Design review of the part built by this model. Coordinates are the model's own, in mm. Face numbers are marked on the shaded views. A direction names the side the tool comes from. Coordinates: 2 decimals unless noted, no trailing zeros. Write each loop counter-clockwise with the first axis right and the second up, starting at its lowest first coordinate (ties: lowest second). Pieces come first, ordered by that corner, then holes. Notation, with made-up numbers: (-14.5, -23) - (-2.5, -23) arc R28 cw to (-2.5, 6) - close; hole circle Ø5 at (65.25, 9). An arc over 180 degrees is marked (long way). One line per item, written item: value.
from build123d import *

# Parameters (mm, degrees)
BOSS_EXTRUDE1_DEPTH      = 22
BOSS_EXTRUDE1_DEPTH_BACK = 22
SKETCH2_W                = 38
SKETCH2_H                = 20
CUT_EXTRUDE1_DEPTH       = 105.423416914
SKETCH3_W                = 7
SKETCH3_H                = 44
BOSS_EXTRUDE2_DEPTH      = 65.5
SKETCH23_R               = 5
SKETCH23_R_2             = 1.2
CUT_EXTRUDE2_DEPTH       = 111.605436123
SKETCH24_W               = 28.5
SKETCH24_H               = 34
CUT_EXTRUDE3_DEPTH       = 90.954502389
SKETCH26_R               = 1.2
SKETCH26_R_2             = 5
SKETCH26_R_3             = 1.45
CUT_EXTRUDE6_DEPTH       = 107.330263801
SKETCH27_W               = 29.7
SKETCH27_H               = 35.2
CUT_EXTRUDE8_DEPTH       = 73.137455597
SKETCH29_W               = 7
SKETCH29_H               = 35
CUT_EXTRUDE10_DEPTH      = 74.468530678
CHAMFER2_SIZE            = 5
FILLET1_START            = -23
FILLET1_DEPTH            = 46
FILLET2_R                = 10
SKETCH30_W               = 35.2
SKETCH30_H               = 20
CUT_EXTRUDE12_DEPTH      = 10


with BuildPart() as part:
    # Sketch1 → Boss-Extrude1 (new, two sides: drawn at the far end of the back side and taken through both)
    with BuildSketch(Plane.XY.offset(-BOSS_EXTRUDE1_DEPTH_BACK)):
        with BuildLine():
            Line((10.25, -60), (10.25, 0))
            ThreePointArc((10.25, 0), (0, -10.25), (-10.25, 0))
            Line((-10.25, 0), (-10.25, -60))
            Line((-10.25, -60), (-10.25, -100))
            Line((-10.25, -100), (10.25, -100))
            Line((10.25, -100), (10.25, -60))
        make_face()
        with BuildLine():
            Line((10.25, 0), (9.2, 0))
            ThreePointArc((9.2, 0), (8.816088231, -0.879772698), (7.91, -1.196620241))
            ThreePointArc((7.91, -1.196620241), (5.656854249, -5.656854249), (1.196620241, -7.91))
            ThreePointArc((1.196620241, -7.91), (1.199154762, -7.954968281), (1.2, -8))
            ThreePointArc((1.2, -8), (-0.045031719, -9.199154762), (-1.196620241, -7.91))
            ThreePointArc((-1.196620241, -7.91), (-5.656854249, -5.656854249), (-7.91, -1.196620241))
            ThreePointArc((-7.91, -1.196620241), (-8.816088231, -0.879772698), (-9.2, 0))
            Line((-9.2, 0), (-10.25, 0))
            ThreePointArc((-10.25, 0), (0, -10.25), (10.25, 0))
        make_face()
        with BuildLine():
            ThreePointArc((7.91, -1.196620241), (7.120227302, -0.816088231), (6.8, 0))
            Line((6.8, 0), (4.2, 0))
            ThreePointArc((4.2, 0), (0, -4.2), (-4.2, 0))
            Line((-4.2, 0), (-6.8, 0))
            ThreePointArc((-6.8, 0), (-7.120227302, -0.816088231), (-7.91, -1.196620241))
            ThreePointArc((-7.91, -1.196620241), (-5.656854249, -5.656854249), (-1.196620241, -7.91))
            ThreePointArc((-1.196620241, -7.91), (0, -6.8), (1.196620241, -7.91))
            ThreePointArc((1.196620241, -7.91), (5.656854249, -5.656854249), (7.91, -1.196620241))
        make_face()
        with BuildLine():
            Line((4.2, 0), (6.8, 0))
            ThreePointArc((6.8, 0), (7.120227302, 0.816088231), (7.91, 1.196620241))
            ThreePointArc((7.91, 1.196620241), (5.656854249, 5.656854249), (1.196620241, 7.91))
            ThreePointArc((1.196620241, 7.91), (0, 6.8), (-1.196620241, 7.91))
            ThreePointArc((-1.196620241, 7.91), (-5.656854249, 5.656854249), (-7.91, 1.196620241))
            ThreePointArc((-7.91, 1.196620241), (-7.120227302, 0.816088231), (-6.8, 0))
            Line((-6.8, 0), (-4.2, 0))
            ThreePointArc((-4.2, 0), (0, 4.2), (4.2, 0))
        make_face()
        with BuildLine():
            ThreePointArc((7.91, 1.196620241), (8.816088231, 0.879772698), (9.2, 0))
            Line((9.2, 0), (10.25, 0))
            ThreePointArc((10.25, 0), (0, 10.25), (-10.25, 0))
            Line((-10.25, 0), (-9.2, 0))
            ThreePointArc((-9.2, 0), (-8.816088231, 0.879772698), (-7.91, 1.196620241))
            ThreePointArc((-7.91, 1.196620241), (-5.656854249, 5.656854249), (-1.196620241, 7.91))
            ThreePointArc((-1.196620241, 7.91), (-0.045031719, 9.199154762), (1.2, 8))
            ThreePointArc((1.2, 8), (1.199154762, 7.954968281), (1.196620241, 7.91))
            ThreePointArc((1.196620241, 7.91), (5.656854249, 5.656854249), (7.91, 1.196620241))
        make_face()
    extrude(amount=BOSS_EXTRUDE1_DEPTH + BOSS_EXTRUDE1_DEPTH_BACK)

    # Sketch2 → Cut-Extrude1 (cut, through all)
    with BuildSketch(Plane.ZY.offset(10.25)):
        with Locations((0, 0.25)):
            Rectangle(SKETCH2_W, SKETCH2_H)
    extrude(amount=-CUT_EXTRUDE1_DEPTH, mode=Mode.SUBTRACT)

    # Sketch3 → Boss-Extrude2 (add)
    with BuildSketch(Plane(origin=(0, -9.75, 0), x_dir=(1, 0, 0), z_dir=(0, 1, 0))):
        with Locations((-13.75, 0)):
            Rectangle(SKETCH3_W, SKETCH3_H)
        with Locations((13.75, 0)):
            Rectangle(SKETCH3_W, SKETCH3_H)
    extrude(amount=-BOSS_EXTRUDE2_DEPTH)

    # Sketch23 → Cut-Extrude2 (cut, through all)
    with BuildSketch(Plane.XY.offset(22)):
        with BuildLine():
            Line((-10.25, -100), (10.25, -100))
            Line((10.25, -100), (10.25, -85))
            ThreePointArc((10.25, -85), (0, -95.25), (-10.25, -85))
            Line((-10.25, -85), (-10.25, -100))
        make_face()
        with Locations((0, -85)):
            Circle(SKETCH23_R)
        with Locations((8, -85)):
            Circle(SKETCH23_R_2)
        with Locations((0, -77)):
            Circle(SKETCH23_R_2)
        with Locations((0, -93)):
            Circle(SKETCH23_R_2)
        with Locations((-8, -85)):
            Circle(SKETCH23_R_2)
    extrude(amount=-CUT_EXTRUDE2_DEPTH, mode=Mode.SUBTRACT)

    # Sketch24 → Cut-Extrude3 (cut, through all)
    with BuildSketch(Plane(origin=(0, -9.75, 0), x_dir=(1, 0, 0), z_dir=(0, 1, 0))):
        Rectangle(SKETCH24_W, SKETCH24_H)
    extrude(amount=-CUT_EXTRUDE3_DEPTH, mode=Mode.SUBTRACT)

    # Sketch26 → Cut-Extrude6 (cut, through all)
    # profile 1 of 5: a face of its own
    with BuildSketch(Plane.XY.offset(22)):
        with BuildLine():
            Line((10.25, -75.25), (14.25, -75.25))
            Line((14.25, -75.25), (14.25, -56.53282359))
            Line((14.25, -56.53282359), (14.25, -56.25))
            Line((14.25, -56.25), (-14.25, -56.25))
            Line((-14.25, -56.25), (-14.25, -56.53282359))
            Line((-14.25, -56.53282359), (-14.25, -75.25))
            Line((-14.25, -75.25), (-10.25, -75.25))
            Line((-10.25, -75.25), (-10.25, -85))
            ThreePointArc((-10.25, -85), (0, -95.25), (10.25, -85))
            Line((10.25, -85), (10.25, -75.25))
        make_face()
        with Locations((-8, -85)):
            Circle(SKETCH26_R, mode=Mode.SUBTRACT)
        with Locations((0, -85)):
            Circle(SKETCH26_R_2, mode=Mode.SUBTRACT)
        with Locations((0, -77)):
            Circle(SKETCH26_R, mode=Mode.SUBTRACT)
        with Locations((0, -93)):
            Circle(SKETCH26_R, mode=Mode.SUBTRACT)
        with Locations((8, -85)):
            Circle(SKETCH26_R, mode=Mode.SUBTRACT)
    # profile 2 of 5: a face of its own
    with BuildSketch(Plane.XY.offset(22)):
        Polygon((-17.25, -75.25), (-14.25, -75.25), (-14.25, -56.53282359), (-14.25, -56.25), (-17.25, -56.25), align=None)
    # profile 3 of 5: a face of its own
    with BuildSketch(Plane.XY.offset(22)):
        Polygon((14.25, -56.53282359), (14.25, -75.25), (17.25, -75.25), (17.25, -56.25), (14.25, -56.25), align=None)
    # profile 4 of 5: a face of its own
    with BuildSketch(Plane.XY.offset(22)):
        with Locations((-11, -53)):
            Circle(SKETCH26_R_3)
    # profile 5 of 5: a face of its own
    with BuildSketch(Plane.XY.offset(22)):
        with Locations((11, -53)):
            Circle(SKETCH26_R_3)
    extrude(amount=-CUT_EXTRUDE6_DEPTH, mode=Mode.SUBTRACT)

    # Sketch27 → Cut-Extrude8 (cut, through all)
    with BuildSketch(Plane.XZ.offset(56.25)):
        Rectangle(SKETCH27_W, SKETCH27_H)
    extrude(amount=-CUT_EXTRUDE8_DEPTH, mode=Mode.SUBTRACT)

    # Sketch29 → Cut-Extrude10 (cut, through all)
    with BuildSketch(Plane(origin=(0, 0, -22), x_dir=(-1, 0, 0), z_dir=(0, 0, -1))):
        with Locations((-13.75, -27.25)):
            Rectangle(SKETCH29_W, SKETCH29_H)
    extrude(amount=-CUT_EXTRUDE10_DEPTH, mode=Mode.SUBTRACT)

    # Chamfer2
    # the kernel refuses this chamfer: 5 mm, written as the material it takes off along each edge
    with BuildSketch(Plane(origin=(-17.25, -56.25, 34.85841494), x_dir=(1, 0, 0), z_dir=(0, 0, -1))) as chamfer2_piece_1:
        Polygon((CHAMFER2_SIZE, 0), (0, -CHAMFER2_SIZE), (0, 0), align=None)
    extrude(amount=69.71682988, mode=Mode.SUBTRACT)

    # Fillet1: read off the stored shape, not the designer's step
    # Fillet1 outline → Fillet1 (cut)
    with BuildSketch(Plane.XY.offset(FILLET1_START)):
        with BuildLine():
            ThreePointArc((10.25, -44.75), (15.312257748, -48.373312231), (17.25, -54.289392014))
            Line((17.25, -54.289392014), (17.25, -44.75))
            Line((17.25, -44.75), (10.25, -44.75))
        make_face()
    extrude(amount=FILLET1_DEPTH, mode=Mode.SUBTRACT)

    # Fillet2
    # the kernel refuses this fillet: 10 mm, written as the material it takes off along each edge
    with BuildSketch(Plane(origin=(-17.25, -9.75, -47), x_dir=(1, 0, 0), z_dir=(0, 0, 1))) as fillet2_piece_1_section:
        with BuildLine():
            CenterArc((FILLET2_R, -FILLET2_R), FILLET2_R, 90, 90)
            Line((0, -FILLET2_R), (0, 0))
            Line((0, 0), (FILLET2_R, 0))
        make_face()
    fillet2_piece_1 = extrude(amount=94, mode=Mode.PRIVATE)
    fillet2_piece_1 = split(fillet2_piece_1, bisect_by=Plane(origin=(-10.25, -9.75, -47), z_dir=(-1, 0, 0)), keep=Keep.TOP, mode=Mode.PRIVATE)
    add(fillet2_piece_1, mode=Mode.SUBTRACT)
    with BuildSketch(Plane(origin=(-17.25, -9.75, -47), x_dir=(1, 0, 0), z_dir=(0, 0, 1))) as fillet2_piece_2_section:
        with BuildLine():
            CenterArc((FILLET2_R, -FILLET2_R), FILLET2_R, 90, 90)
            Line((0, -FILLET2_R), (0, 0))
            Line((0, 0), (FILLET2_R, 0))
        make_face()
    fillet2_piece_2 = extrude(amount=94, mode=Mode.PRIVATE)
    fillet2_piece_2 = split(fillet2_piece_2, bisect_by=Plane(origin=(-17.25, -9.75, -19), z_dir=(0, 0, 1)), keep=Keep.TOP, mode=Mode.PRIVATE)
    fillet2_piece_2 = split(fillet2_piece_2, bisect_by=Plane(origin=(-17.25, -9.75, 19), z_dir=(0, 0, -1)), keep=Keep.TOP, mode=Mode.PRIVATE)
    add(fillet2_piece_2, mode=Mode.SUBTRACT)

    # Sketch30 → Cut-Extrude12 (cut)
    with BuildSketch(Plane.ZY.offset(17.25)):
        with Locations((0, -23.250769276)):
            Rectangle(SKETCH30_W, SKETCH30_H)
    extrude(amount=-CUT_EXTRUDE12_DEPTH, mode=Mode.SUBTRACT)


solid = part.part
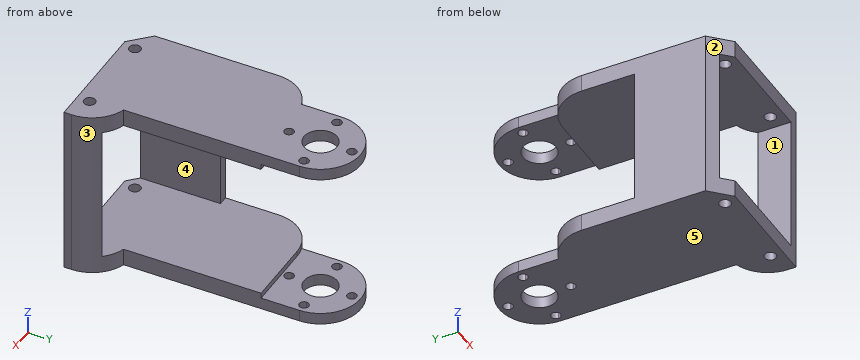
1. Insertion check: pin 1 Ø11 at (x, y) = (0, 0) entering from +Z; pin 2 Ø1 at (x, y) = (12.5, -41) entering from +Z (3 decimals); pin 3 Ø4 at (y, z) = (-36, 1) entering from +X; pin 4 Ø5 at (y, z) = (-33, 19) entering from +X. Each pin has a flat end and moves straight along its axis. Give the tip position at first contact, or say it passes through.
Answer block:
pin 1: stops at z = 22
pin 2: passes through
pin 3: stops at x = -14.85
pin 4: stops at x = 10.25
2. Consider section D-D, the plane x = 0. Give the number of separate pieces and of enclosed holes in the cut face, then the cut area to 3 significant figures.
Answer block:
separate pieces: 8
enclosed holes: 0
area: 450 mm^2
3. Mouldability with a two-part tool opening along X and no side actions: class the marked faces 1, 2 and 3 as released by +X, released by -X, zero draft, split by the parting line, or undercut.
Answer block:
face 1: undercut
face 2: released by -X
face 3: released by +X
4. Consider section C-C, the plane x = -11. Write out the cut boundary in (y, z), then the cut area to 3 significant figures.
Answer block:
outline: (-56.25, -22) - (-54.45, -22) - (-54.45, -17.6) - (-56.25, -17.6) - close; (-56.25, 17.6) - (-54.45, 17.6) - (-54.45, 22) - (-56.25, 22) - close; (-51.55, -22) - (-10.48, -22) - (-10.48, -17.6) - (-51.55, -17.6) - close; (-51.55, 17.6) - (-10.48, 17.6) - (-10.48, 22) - (-51.55, 22) - close
area: 377 mm^2
5. For the marked faces 4 and 5, list the 3-axis set-ups (+Z, -Z, +X, -X, +Y, -Y) from which the entire face can be reached by the end or side of a thin tool; tool diameter is ignored.
Answer block:
face 4: +Y, -Y
face 5: -Z, +X, -X, +Y, -Y
6. Wall thickness on line 1 along Z through (x, y) = (-8.5, -3.5); line 2 along Z through (x, y) = (-5, -20); line 3 along X through (y, z) = (-35.5, -1): over which ranges is each line inside the solid? List them lowest first.
Answer block:
line 1: z = -22 to -19, 19 to 22
line 2: z = -22 to -17.6, 17.6 to 22
line 3: x = -17.25 to -14.85
7. Consider section B-B, the plane y = -29. Write out the cut boundary in (x, z).
Answer block:
outline: (-17.25, -22) - (10.25, -22) - (10.25, -17.6) - (-17.25, -17.6) - close; (-17.25, 17.6) - (10.25, 17.6) - (10.25, 22) - (-17.25, 22) - close
8. Consider section A-A, the plane z = -15.5. Write out the cut boundary in (x, y), then the cut area to 3 significant figures.
Answer block:
outline: (-17.25, -51.25) - (-14.85, -53.65) - (-14.85, -33.25) - (-17.25, -33.25) - close; (14.85, -56.25) - (17.25, -56.25) - (17.25, -54.29) arc R10 ccw to (14.85, -47.79) - close
area: 61.5 mm^2
